Verification items for this drawing (mm, ordinates from the low corner). A direction names the side the tool comes from. Coordinates: 2 decimals unless noted, no trailing zeros. Write each loop counter-clockwise with the first axis right and the second up, starting at its lowest first coordinate (ties: lowest second). Pieces come first, ordered by that corner, then holes. Notation, with made-up numbers: (-22, -21) -> (11, -21) arc R25 cw to (11, 11) -> close; hole circle Ø4 at (-15, 78). An arc over 180 degrees is marked (long way). One line per item, written item: value. Start each with the question number.
1) Set-up check for the marked faces 1 and 2: record each of +Z, -Z, +X, -X, +Y, -Y from which the full face is reachable in a straight line by a thin tool's end or side.
2) Sectioned sample at A-A on y = 37. Enter the section's corners in (x, z) (1 decimal), plus the area to 3 significant figures.
3) Gauge pin test, flat ends, axial feed: P1, Ø8, axis at x = 37.5, z = 54.5, coming from the +Y side; P2, Ø1, axis at y = 32.5, z = 53.5, coming from the +X side; P3, Ø1, axis at y = 16.5, z = 12, coming from the -X side; P4, Ø2, axis at y = 6, z = 39, coming from the -X side. Record the tip position at first contact, or that the pin passes through.
4) Scan lines: line 1 along Y through (x, z) = (47, 20.5); line 2 along X through (y, z) = (20.5, 37); line 3 along X through (y, z) = (23.5, 41) (1 decimal). Record each from-to range of solid material in increasing order. Write a range as [from, to].
5) Sectioned sample at B-B on y = 29.5. Enter the section's corners in (x, z).
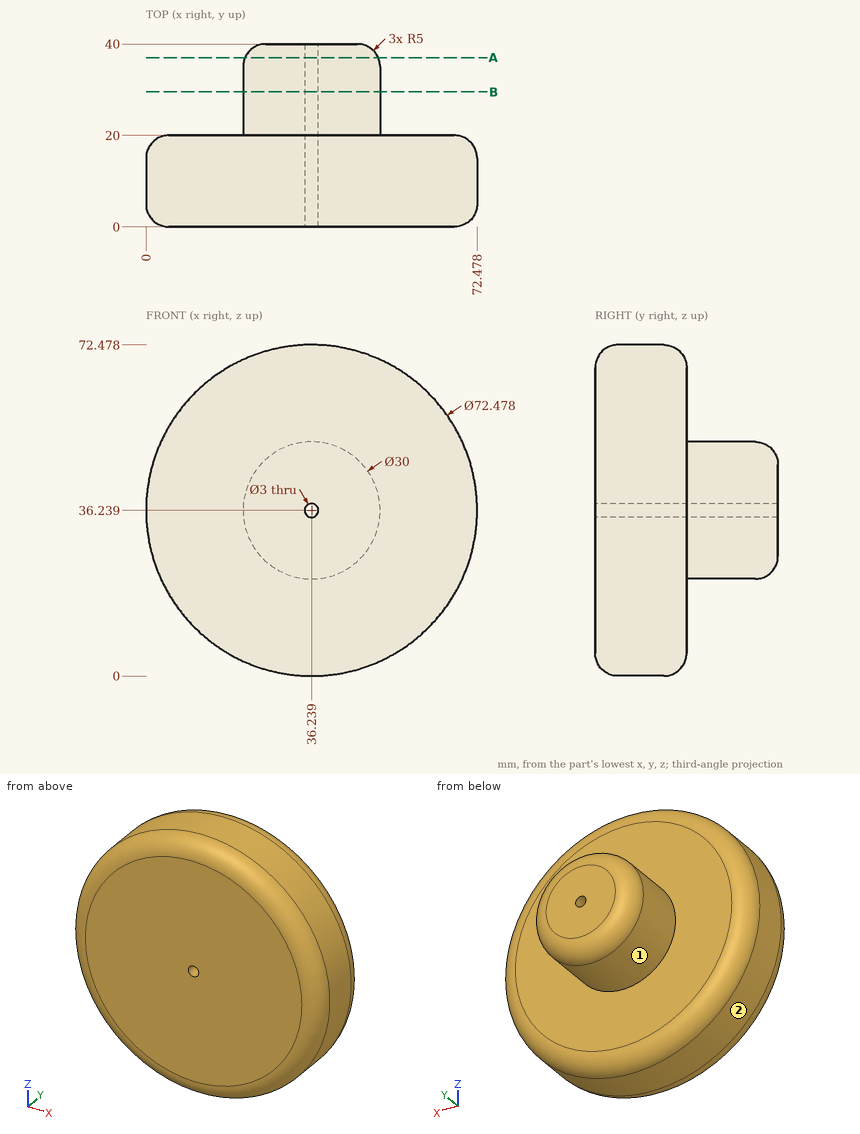
Answers:
1. face 1: +Y
1. face 2: +Y, -Y
2. outline: circle Ø29.2 at (36.2, 36.2); hole circle Ø3 at (36.2, 36.2)
2. area: 661 mm2
3. P1: stops at y = 37.54
3. P2: passes through
3. P3: stops at x = 9.12
3. P4: stops at x = 0.04
4. line 1: y = [0, 20]
4. line 2: x = [21.26, 34.95], [37.53, 51.22]
4. line 3: x = [22, 50.5]
5. outline: circle Ø30 at (36.24, 36.24); hole circle Ø3 at (36.24, 36.24)
